```python
from build123d import *

# Parameters (mm, degrees)
F1_DEPTH = 25.4


with BuildPart() as f1:
    # F0 (on Top) → F1 (new body)
    with BuildSketch(Plane.XY):
        with BuildLine():
            ThreePointArc((-105.059527, 114.809577), (-12.430289, 52.195551), (-33.424245, -57.622234))
            ThreePointArc((-33.424245, -57.622234), (-2.611057, -42.983897), (15.07293, -13.811819))
            ThreePointArc((15.07293, -13.811819), (18.193999, 44.569559), (-7.210166, 97.226513))
            ThreePointArc((-7.210166, 97.226513), (-31.495036, 117.82512), (-61.715451, 127.864246))
            ThreePointArc((-61.715451, 127.864246), (-84.379276, 124.629841), (-105.059527, 114.809577))
        make_face()
    extrude(amount=F1_DEPTH)


solid = f1.part
```
Build history of the part. All positions in model axes, mm. Round coordinates to 2 decimals unless told otherwise and drop trailing zeros. Write each loop counter-clockwise with the first axis right and the second up, starting at its lowest first coordinate (ties: lowest second). Pieces come first, ordered by that corner, then holes. Notation, with made-up numbers: (48.5, 61) - (65.5, 61) arc R18 ccw to (65.5, 78) - close; hole circle Ø1 at (68.25, 69.5). An arc over 180 degrees is marked (long way). Write each question's results on one line, items separated by ' | '. Start each with the question number.
Item 1: Drop flat-ended pins along their axis: P1, Ø3, axis at y = -10.5, z = 4, coming from the +X side (3 decimals); P2, Ø8, axis at x = 0.5, z = 11, coming from the +Y side; P3, Ø1, axis at y = 73.5, z = 19, coming from the +X side. Give the stop position or say it passes through.
Item 2: Mould opens along Y. For faces 1 (the face through (-31.1, 117.6, 12.5)), 2 (the face through (-13.08, 53.72, 12.52)), 3 (the face through (-10, 56, 25.4)) say: pulls with the +Y half, pulls with the -Y half, needs draft (parallel to the pull), parting line crosses it, or undercut.
Item 3: Wall check: L1, parallel to Y at x = -14.5, z = 9.5; L2, parallel to Y at x = -77.5, z = 13.5; L3, parallel to Y at x = -74.5, z = 7. Give the ranges that are in metal, low to high. Write a range as [from, to].
Item 4: Saw through at B-B (z = 14.75). Write the cut outline in (x, y), and give its area (3 significant figures).
Item 5: Saw through at C-C (y = 104). Write the cut outline in (x, z).
Item 6: Saw through at A-A (x = -29.5). Write the cut outline in (y, z), and give its area (3 significant figures).
Item 7: Saw through at D-D (x = -13.5). Write the cut outline in (y, z).
Results are:
1) P1: stops at x = 16.475 | P2: stops at y = 92.6 | P3: stops at x = 8.58
2) face 1: pulls with the +Y half | face 2: undercut | face 3: needs draft
3) L1: y = [-51.33, -30.41], [56.85, 105.2] | L2: y = [110.66, 126.36] | L3: y = [109.73, 126.9]
4) outline: (-105.06, 114.81) arc R101.6 cw to (-33.42, -57.62) arc R59.42 ccw to (15.07, -13.81) arc R117.49 ccw to (-7.21, 97.23) arc R83.71 ccw to (-61.72, 127.86) arc R76.2 ccw to start | area: 5,630 mm²
5) outline: (-60.64, 0) - (-13.28, 0) - (-13.28, 25.4) - (-60.64, 25.4) - close
6) outline: (-56.88, 0) - (-53.35, 0) - (-53.35, 25.4) - (-56.88, 25.4) - close; (79.78, 0) - (116.67, 0) - (116.67, 25.4) - (79.78, 25.4) - close | area: 1,030 mm²
7) outline: (-50.79, 0) - (-28.24, 0) - (-28.24, 25.4) - (-50.79, 25.4) - close; (54.68, 0) - (104.22, 0) - (104.22, 25.4) - (54.68, 25.4) - close
